Verification items for this drawing (mm, ordinates from the low corner). A direction names the side the tool comes from. Give positions to 0.01 mm unless a question says otherwise; leave off trailing zeros. Order: outer loops, then holes, each group sorted by start corner. A loop starts at its lowest first (then second) coordinate and runs counter-clockwise, first axis right, second up.
(1) Scan lines: L1, parallel to X at y = 23, z = 10; L2, parallel to Z at x = 18, y = 4; L3, parallel to Z at x = 10, y = 32. Record each from-to range of solid material in increasing order.
(2) Sectioned sample at A-A on y = 7. Record the cut outline in (x, z).
(3) Gauge pin test, flat end, axial feed: pin 1 (6.5 mm diameter, centred on x = 10.5, z = 53.5, fed in from -Y). Record the tip position at first contact, or that the pin passes through.
(4) Mould release check, pull along Z, two halves, no side actions. Record for the marked faces 3, 4 and 5: pulls with the +Z half, pulls with the -Z half, needs draft (parallel to the pull), parting line crosses it, or undercut.
(5) Access from +Z, -Z, +X, -X, +Y, -Y to the whole of each face (thin tool, end or side, straight path). Record for the marked faces 1 and 2.
(6) Sectioned sample at D-D on y = 39. Record the cut outline in (x, z).
(7) Sectioned sample at B-B on z = 10. Record the cut outline in (x, y).
(8) Sectioned sample at C-C on x = 7. Record the cut outline in (y, z).
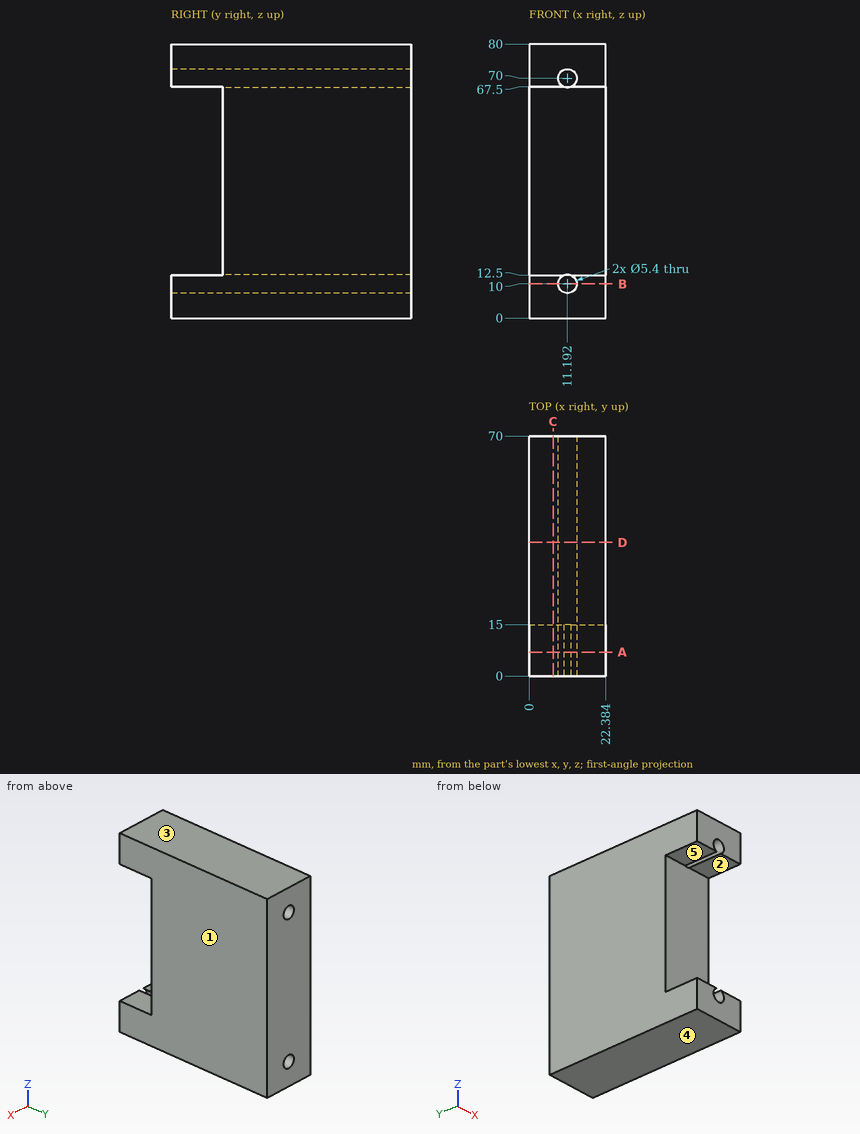
Ans:
1. L1: x = 0 to 8.49, 13.89 to 22.38
1. L2: z = 0 to 12.5, 67.5 to 80
1. L3: z = 0 to 7.58, 12.42 to 67.58, 72.42 to 80
2. outline: (0, 0) - (22.38, 0) - (22.38, 12.5) - (12.21, 12.5) arc R2.7 cw (long way) to (10.17, 12.5) - (0, 12.5) - close; (0, 67.5) - (10.17, 67.5) arc R2.7 cw (long way) to (12.21, 67.5) - (22.38, 67.5) - (22.38, 80) - (0, 80) - close
3. pin 1: stops at y = 15
4. face 3: pulls with the +Z half
4. face 4: pulls with the -Z half
4. face 5: undercut
5. face 1: +Z, -Z, +X, +Y, -Y
5. face 2: +X, -X, -Y
6. outline: (0, 0) - (22.38, 0) - (22.38, 80) - (0, 80) - close; hole circle Ø5.4 at (11.19, 10); hole circle Ø5.4 at (11.19, 70)
7. outline: (0, 0) - (8.49, 0) - (8.49, 70) - (0, 70) - close; (13.89, 0) - (22.38, 0) - (22.38, 70) - (13.89, 70) - close
8. outline: (0, 0) - (70, 0) - (70, 80) - (0, 80) - (0, 67.5) - (15, 67.5) - (15, 12.5) - (0, 12.5) - close
